Verification items for the finished model (mm, model axes). A direction names the side the tool comes from. Round coordinates to 2 decimals unless told otherwise and drop trailing zeros. Order: outer loops, then holes, each group sorted by start corner. A loop starts at its lowest first (then second) coordinate and runs counter-clockwise, first axis right, second up. Notation, with made-up numbers: M -15.75,86.25 L 30.25,86.25 A16 ccw 30.25,117.25 Z; hole C 63.5,40 d7. An arc over 180 degrees is marked long. Use CSV: the item, a comma, the result in double quotes. Start each with the question number.
Q1. Set-up check for faces 3 (the face through (0, 156, -14)), 4 (the face through (0.54, 74.94, 2.44)): record each of +Z, -Z, +X, -X, +Y, -Y from which the full face is reachable in a straight line by a thin tool's end or side.
Q2. Scan lines: line 1 (Y direction, x = -0.35, z = -6.25); line 2 (Z direction, x = -0.4, y = 8.5); line 3 (Z direction, x = 0.6, y = 146). Record each from-to range of solid material in increasing order.
Q3. Mould release check, pull along X, two halves, no side actions. Record for faces 1 (the face through (0.33, 153.52, -8.93)), 2 (the face through (0, 0, 0)): +X half, -X half, draft (parallel to the pull), parting line (faces both ways), or undercut.
Q4. Gauge pin test, flat ends, axial feed: pin 1 Ø2 at (y, z) = (92.5, -1.5) entering from -X; pin 2 Ø1.5 at (x, z) = (1, -7) entering from +Y; pin 3 Ø1.5 at (x, z) = (0, -7) entering from -Y. Record the tip position at first contact, or that the pin passes through.
Q5. Sectioned sample at A-A (x = 0). Enter the section's corners in (y, z), and give its area (3 significant figures).
Q6. Sectioned sample at B-B (y = 131). Enter the section's corners in (x, z), and give its area (3 significant figures).
Autodesk Inventor part; units mm, degrees
ref_plane "YZ Plane" through (0, 0, 0) normal (1, 0, 0) x (0, 1, 0)
ref_plane "XZ Plane" through (0, 0, 0) normal (0, 1, 0) x (-1, 0, 0)
ref_plane "XY Plane" through (0, 0, 0) normal (0, 0, 1) x (1, 0, 0)
sketch "Sketch1" plane through (0, 0, 0) normal (0, 1, 0) x (-1, 0, 0)
  circle A0 centre (0, 0) radius 2.5
  dimension "d0" = 5
extrude "Extrusion1" add sketch "Sketch1" along normal blind 152
sketch "Sketch2" plane through (0, 0, 0) normal (1, 0, 0) x (0, 1, 0)
  arc A0 (148.2919, -2.5) -> (156, -4) centre (152, -4) ccw construction
  line L0 (152, -2.5) -> (152, 2.5)
  line L1 (0, -2.5) -> (152, -2.5)
  line L2 (0, 2.5) -> (152, 2.5)
  arc A1 (152, 0) -> (148.2919, -2.5) centre (152, -4) ccw construction
  arc A2 (155.7081, -2.5) -> (152, 0) centre (152, -4) ccw
  line L3 (152, 0) -> (159.1444, 0) construction
  line L4 (152, -4) -> (156, -4) construction
  arc A3 (156, -4) -> (155.7081, -2.5) centre (152, -4) ccw
  point P0 (0, 0)
  dimension "d3" = 8
sketch "Sketch3" plane through (0, 152, 0) normal (0, 1, 0) x (1, 0, 0)
  circle A0 centre (0, 0) radius 2.5
sweep "Sweep1" add profiles "Sketch3" path "Sketch2" path curves A2 A3
sketch "Sketch4" plane through (0, 156, -4) normal (0, 0, -1) x (-1, 0, 0)
  circle A0 centre (0, 0) radius 2.5
  point P0 (0, -156)
extrude "Extrusion2" add sketch "Sketch4" along normal blind 10
properties part number "Eje" material "Stainless Steel"
Verdict:
1,face 3,"-Z, +X, -X, +Y, -Y"
1,face 4,"-Y"
2,line 1,"y = 153.52 to 158.48"
2,line 2,"z = -2.47 to 2.47"
2,line 3,"z = -2.43 to 2.43"
3,face 1,"parting line"
3,face 2,"draft"
4,pin 1,"stops at x = -2.45"
4,pin 2,"stops at y = 158.49"
4,pin 3,"stops at y = 153.5"
5,outline,"M 0,-2.5 L 152,-2.5 A1.5 cw 153.39,-3.44 A1.5 cw 153.5,-4 L 153.5,-14 L 158.5,-14 L 158.5,-4 A6.5 ccw 158.03,-1.56 A6.5 ccw 152,2.5 L 0,2.5 Z"
5,area,"841 mm²"
6,outline,"C 0,0 d5"
6,area,"19.6 mm²"
